The listing builds one solid part. Answer for the finished solid, in the listing's coordinates (mm). A direction names the side the tool comes from. Give positions to 0.01 mm unless a question says otherwise; leave off trailing zeros. Loops run counter-clockwise (first coordinate to the right, second up) from the corner with the lowest first, then second, coordinate; pieces in that order, holes last. Notation, with made-up numbers: (-37, 34.25) - (-17, 34.25) arc R18 cw to (-17, 60.25) - close; hole circle Ø3 at (53, 60.5). An arc over 180 degrees is marked (long way). Answer as CSV lines item,"result". Start each with the question number.
1) A cutting plane is placed at B-B (z = 848). Determine the outline of the cut face in (x, y), and give its area (4 significant figures).
2) For a pull along Y with two mould halves and no side action, classify faces 1 (the face through (118, -135, 649)), 2 (the face through (100, -86, 49)), 3 (the face through (118, -132.5, 647)) as pulls with the +Y half, pulls with the -Y half, needs draft (parallel to the pull), parting line crosses it, or undercut.
3) A cutting plane is placed at A-A (y = -55). Determine the outline of the cut face in (x, z), and give its area (3 significant figures).
4) For faces 4 (the face through (51, -35, 51)), 5 (the face through (49, -37.5, 55)), 6 (the face through (237.5, 2, 766)), determine the directions among +Z, -Z, +X, -X, +Y, -Y from which every point of the face is accessible in a straight line to the end or side of a thin tool.
5) A cutting plane is placed at D-D (y = -6). Determine the outline of the cut face in (x, z), and give its area (3 significant figures).
6) Find the intervals of material crossed by line 1 along X through (y, z) = (-2, 728.5); line 2 along Y through (x, z) = (137.5, 997); line 3 along X through (y, z) = (-111.5, 42), in increasing order.
7) A cutting plane is placed at C-C (x = 215). Determine the outline of the cut face in (y, z).
8) Flat-ended cylindrical pins translate along their axes: pin 1 (5.5 mm diameter, centred on x = 156.5, z = 1048.5, fed in from +Y); pin 2 (12 mm diameter, centred on y = -37, z = 294.5, fed in from -X); pin 3 (1.5 mm diameter, centred on x = 136, z = 1043, fed in from +Y); pin 4 (8 mm diameter, centred on x = 67, z = 5.5, fed in from -Y). Find the tip coordinate at first contact, or state that the pin passes through.
```python
from build123d import *

# Parameters (mm, degrees)
F0_W        = 100
F0_H        = 100
F1_DEPTH    = 135
F3_DEPTH    = 240
F4_T        = 2.5
F4_T3_DEPTH = 105
F4_T5_DEPTH = 105
F6_DEPTH    = 98.5
F7_W        = 235
F7_H        = 5
F8_DEPTH    = 2.5
F9_DEPTH    = 269


# Not quite as in the source:
# - a shell that OpenCascade refuses in one call is made with other operations: the cavity is built on its own and cut out


with BuildPart() as f1:
    # F0 (on Front) → F1 (new body, symmetric)
    with BuildSketch(Plane.XZ):
        Polygon((0, 500), (0, 100), (100, 100), (240, 500), (240, 1050), (0, 1050), align=None)
        with Locations((50, 50)):
            Rectangle(F0_W, F0_H)
    extrude(amount=F1_DEPTH, both=True)

    # F2 (on face) → F3 (cut)
    with BuildSketch(Plane.YZ.offset(240)):
        Polygon((135, 0), (135, 500), (-35, 100), (-35, 0), align=None)
    extrude(amount=-F3_DEPTH, mode=Mode.SUBTRACT)

    # F4: shell of thickness 2.5, made by hand


with BuildPart() as f4_core1:
    # F4_t2: copy of F1
    add(f1.part)

    # the walls: a layer under each face that stays
    f4_faces = [f4_core1.faces().sort_by_distance(p)[0] for p in [
        (0, 0, 525),
        (120, -135, 525),
        (100, -85, 50),
        (50, -35, 50),
        (120, 50, 300),
        (120, 135, 775),
        (170, 0, 300),
        (240, 0, 775),
    ]]
    thicken(f4_faces, amount=-F4_T, mode=Mode.SUBTRACT)

    # F4_s4 → F4_t3 (cut)
    with BuildSketch(Plane.XZ.offset(32.5)):
        Polygon((100.0485964589, 99.9917412394), (97.5, 100), (97.5, 100.4248643216), (97.6403541091, 100.8258760618), align=None)
    extrude(amount=F4_T3_DEPTH, mode=Mode.SUBTRACT)

    # F4_s6 → F4_t5 (cut)
    with BuildSketch(Plane.YZ.offset(-2.5)):
        Polygon((-34.951991727, 99.990221484), (-37.5, 100), (-37.5, 100.5092099447), (-37.3008272961, 100.9778516009), align=None)
    extrude(amount=F4_T5_DEPTH, mode=Mode.SUBTRACT)


with BuildPart() as f1_1:
    add(f1.part)

    # what is left inside the walls is the cavity
    f4_cavity = [f4_core1.part.solids().sort_by_distance(p)[0] for p in [
        (2.525, 44.166667, 525),
    ]]
    add(f4_cavity, mode=Mode.SUBTRACT)

    # F5 (on face) → F6 (cut)
    with BuildSketch(Plane.XZ.offset(135)):
        Polygon((1.5, 5), (1.5, 0), (98.5, 0), (98.5, 5), (99.5, 5), (99.5, 10), (0.5, 10), (0.5, 5), align=None)
    extrude(amount=-F6_DEPTH, mode=Mode.SUBTRACT)

    # F7 (on face) → F8 (cut)
    with BuildSketch(Plane(origin=(0, 135, 0), x_dir=(-1, 0, 0), z_dir=(0, 1, 0))):
        with Locations((-120, 1047.5)):
            Rectangle(F7_W, F7_H)
    extrude(amount=-F8_DEPTH, mode=Mode.SUBTRACT)

    # F7 (on face) → F9 (cut)
    with BuildSketch(Plane(origin=(0, 135, 0), x_dir=(-1, 0, 0), z_dir=(0, 1, 0))):
        Polygon((-2.5, 1045), (-237.5, 1045), (-239, 1045), (-239, 1040), (-1, 1040), (-1, 1045), align=None)
    extrude(amount=-F9_DEPTH, mode=Mode.SUBTRACT)


solid = f1_1.part
```
Ans:
1,outline,"(0, -135) - (240, -135) - (240, 135) - (0, 135) - close; hole (2.5, -132.5) - (237.5, -132.5) - (237.5, 132.5) - (2.5, 132.5) - close"
1,area,"2,525 mm2"
2,face 1,"pulls with the -Y half"
2,face 2,"needs draft"
2,face 3,"undercut"
3,outline,"(0, 0) - (1.5, 0) - (1.5, 5) - (0.5, 5) - (0.5, 10) - (2.5, 10) - (2.5, 1040) - (1, 1040) - (1, 1045) - (2.5, 1045) - (2.5, 1050) - (0, 1050) - close; (97.5, 10) - (99.5, 10) - (99.5, 5) - (98.5, 5) - (98.5, 0) - (100, 0) - (100, 100) - (240, 500) - (240, 1050) - (237.5, 1050) - (237.5, 1045) - (239, 1045) - (239, 1040) - (237.5, 1040) - (237.5, 500.42) - (97.5, 100.42) - close"
3,area,"5,260 mm2"
4,face 4,"-Z, +X, -X, +Y"
4,face 5,"+Z, -Z"
4,face 6,"+Z"
5,outline,"(0, 168.24) - (123.88, 168.24) - (240, 500) - (240, 1050) - (237.5, 1050) - (237.5, 1045) - (239, 1045) - (239, 1040) - (237.5, 1040) - (237.5, 500.42) - (123.47, 174.63) - (2.5, 174.63) - (2.5, 1040) - (1, 1040) - (1, 1045) - (2.5, 1045) - (2.5, 1050) - (0, 1050) - close"
5,area,"5,210 mm2"
6,line 1,"0 to 2.5, 237.5 to 240"
6,line 2,"-135 to -132.5, 132.5 to 135"
6,line 3,"0 to 2.5, 97.5 to 100"
7,outline,"(-135, 428.57) - (104.64, 428.57) - (135, 500) - (135, 1040) - (132.5, 1040) - (132.5, 500.51) - (105.14, 436.14) - (-132.5, 436.14) - (-132.5, 1040) - (-134, 1040) - (-134, 1045) - (-132.5, 1045) - (-132.5, 1050) - (-135, 1050) - close"
8,pin 1,"y = -132.5"
8,pin 2,"x = 0"
8,pin 3,"y = -134"
8,pin 4,"y = -36.5"
